Can you work these out from the model? Positions are in its coordinate system, mm. A direction names the side the tool comes from. Give positions to 0.01 mm unless a question says otherwise; leave off trailing zeros. Write each loop counter-clockwise with the first axis right and the second up, starting at its lowest first coordinate (ties: lowest second). Pieces come first, ordered by that corner, then holes.
from build123d import *

# Parameters (mm, degrees)
SKETCH_3_W          = 50
SKETCH_3_H          = 30
EXTRUDE_1_DEPTH     = 100
SKETCH_4_W          = 20
SKETCH_4_H          = 41
CUT_EXTRUDE_1_DEPTH = 37
SKETCH_5_W          = 19
SKETCH_5_H          = 7
CUT_EXTRUDE_2_DEPTH = 8
SKETCH_6_W          = 7
SKETCH_6_H          = 7
CUT_EXTRUDE_3_DEPTH = 29
SKETCH_8_W          = 9
SKETCH_8_H          = 10
CUT_EXTRUDE_4_DEPTH = 61
SKETCH_9_W          = 10
SKETCH_9_H          = 10
CUT_EXTRUDE_5_DEPTH = 5
FILLET_1_R          = 5
SKETCH_10_R         = 3
CUT_EXTRUDE_6_DEPTH = 5


with BuildPart() as part:
    # 草圖3 → 填料-伸長1 (new body)
    with BuildSketch(Plane(origin=(0, 0, 0), x_dir=(1, 0, 0), z_dir=(0, 1, 0))):
        with Locations((8, 3)):
            Rectangle(SKETCH_3_W, SKETCH_3_H)
    extrude(amount=EXTRUDE_1_DEPTH)

    # 草圖4 → 除料-伸長1 (cut)
    with BuildSketch(Plane(origin=(33, 0, 0), x_dir=(0, 0, -1), z_dir=(1, 0, 0))):
        with Locations((3, 59.5)):
            Rectangle(SKETCH_4_W, SKETCH_4_H)
    extrude(amount=-CUT_EXTRUDE_1_DEPTH, mode=Mode.SUBTRACT)

    # 草圖5 → 除料-伸長2 (cut)
    with BuildSketch(Plane(origin=(33, 0, 0), x_dir=(0, 0, -1), z_dir=(1, 0, 0))):
        with Locations((3, 83.5)):
            Rectangle(SKETCH_5_W, SKETCH_5_H)
        with Locations((3, 35.5)):
            Rectangle(SKETCH_5_W, SKETCH_5_H)
    extrude(amount=-CUT_EXTRUDE_2_DEPTH, mode=Mode.SUBTRACT)

    # 草圖6 → 除料-伸長3 (cut)
    with BuildSketch(Plane(origin=(25, 0, 0), x_dir=(0, 0, -1), z_dir=(1, 0, 0))):
        with Locations((3, 83.5)):
            Rectangle(SKETCH_6_W, SKETCH_6_H)
    extrude(amount=-CUT_EXTRUDE_3_DEPTH, mode=Mode.SUBTRACT)

    # 草圖8 → 除料-伸長4 (cut)
    with BuildSketch(Plane(origin=(0, 100, 0), x_dir=(1, 0, 0), z_dir=(0, 1, 0))):
        with Locations((-7.5, 3)):
            Rectangle(SKETCH_8_W, SKETCH_8_H)
    extrude(amount=-CUT_EXTRUDE_4_DEPTH, mode=Mode.SUBTRACT)

    # 草圖9 → 除料-伸長5 (cut)
    with BuildSketch(Plane.ZY.offset(17)):
        with Locations((-3, 44)):
            Rectangle(SKETCH_9_W, SKETCH_9_H)
    extrude(amount=-CUT_EXTRUDE_5_DEPTH, mode=Mode.SUBTRACT)

    # 圓角1
    fillet_1_edges = [part.edges().sort_by_distance(p)[0] for p in [
        (-12, 49, -3),
    ]]
    fillet(fillet_1_edges, radius=FILLET_1_R - 0.0001)  # a hair under: the kernel refuses the full size

    # 草圖10 → 除料-伸長6 (cut)
    with BuildSketch(Plane.ZY.offset(17)):
        with Locations((-2.038456717, 71)):
            Circle(SKETCH_10_R)
    extrude(amount=-CUT_EXTRUDE_6_DEPTH, mode=Mode.SUBTRACT)


solid = part.part
(1) Imagine slicing it at D-D, the plane z = -1. Give the number of separate pieces and of enclosed holes in the cut face, plus the area to 3 significant figures.
Returned:
separate pieces: 4
enclosed holes: 0
area: 2,580 mm2
(2) Imagine slicing it at B-B, the plane x = 2. Write out the boundary of the cut face in (y, z), plus the area to 3 significant figures.
Returned:
outline: (0, -18) - (100, -18) - (100, 12) - (0, 12) - close; hole (39, -13) - (80, -13) - (80, -6.5) - (87, -6.5) - (87, 0.5) - (80, 0.5) - (80, 7) - (39, 7) - close
area: 2,130 mm2
(3) Will this pin go through, and if not, where does the flat tip stop? P1, Ø3, axis at y = 84.5, z = 2, coming from the +X side.
Returned:
P1: stops at x = 25
(4) Imagine slicing it at C-C, the plane y = 94. Write out the boundary of the cut face in (x, z).
Returned:
outline: (-17, -18) - (33, -18) - (33, 12) - (-17, 12) - close; hole (-12, -8) - (-3, -8) - (-3, 2) - (-12, 2) - close
(5) Imagine slicing it at A-A, the plane y = 71. Write out the boundary of the cut face in (x, z), plus the area to 3 significant figures.
Returned:
outline: (-17, -18) - (33, -18) - (33, -13) - (-4, -13) - (-4, -8) - (-12, -8) - (-12, -5.04) - (-17, -5.04) - close; (-17, 0.96) - (-12, 0.96) - (-12, 2) - (-4, 2) - (-4, 7) - (33, 7) - (33, 12) - (-17, 12) - close
area: 650 mm2
(6) If I drill on L1, parallel to Z at x = -9.5, y = 86.5; L2, parallel to Y at x = 8.5, z = -11; L3, parallel to Z at x = 18, y = 48.5, over which ranges is the centre line in solid material (lowest first)?
Returned:
L1: z = -18 to -8, 2 to 12
L2: y = 0 to 39, 80 to 100
L3: z = -18 to -13, 7 to 12
(7) If we mould it in two halves opening along Y, with no side actions, what happens to faces 3 (the face through (19, 87, -3)), 4 (the face through (8, 0, -3)), 5 (the face through (8, 49, -18))? For each: +Y half, -Y half, draft (parallel to the pull), parting line (faces both ways), or undercut.
Returned:
face 3: undercut
face 4: -Y half
face 5: draft
(8) For faces 1 (the face through (-17, 49.3, -2.8)), 2 (the face through (-13, 51, -3)), which set-ups out of +Z, -Z, +X, -X, +Y, -Y let a thin tool reach every point of the face, with its end or its side?
Returned:
face 1: +Z, -Z, -X, +Y, -Y
face 2: +X
